```python
from build123d import *

# Parameters (mm, degrees)
CROQUIS1_R              = 5
SALIENTE_EXTRUIR1_DEPTH = 40
CORTAR_EXTRUIR2_DEPTH   = 10
CORTAR_EXTRUIR4_DEPTH   = 20
CROQUIS6_R              = 12.2
CORTAR_EXTRUIR6_DEPTH   = 63
CORTAR_EXTRUIR9_DEPTH   = 30
CROQUIS8_W              = 12.2
CROQUIS8_H              = 11.6
CORTAR_EXTRUIR10_DEPTH  = 66
CORTAR_EXTRUIR11_REACH  = 151.27
CROQUIS9_W              = 11.6
CROQUIS9_H              = 11.6
CHAFL_N1_SIZE           = 10


with BuildPart() as part:
    # Croquis1 → Saliente-Extruir1 (new body)
    with BuildSketch(Plane.XY):
        with BuildLine():
            Line((106.972889038, 33), (-43.027110962, 33))
            ThreePointArc((-43.027110962, 33), (-76.027110962, 0), (-43.027110962, -33))
            Line((-43.027110962, -33), (106.972889038, -33))
            ThreePointArc((106.972889038, -33), (139.972889038, 0), (106.972889038, 33))
        make_face()
        with Locations((106.972889038, 0)):
            Circle(CROQUIS1_R, mode=Mode.SUBTRACT)
    extrude(amount=SALIENTE_EXTRUIR1_DEPTH)

    # Croquis1<4> → Cortar-Extruir2 (cut)
    with BuildSketch(Plane.XY):
        with BuildLine():
            Line((-41.509889959, -1.303088803), (-41.509889959, 1.303088803))
            ThreePointArc((-41.509889959, 1.303088803), (-45.027110962, 0), (-41.509889959, -1.303088803))
        make_face()
    extrude(amount=CORTAR_EXTRUIR2_DEPTH, mode=Mode.SUBTRACT)

    # Croquis5 → Cortar-Extruir4 (cut)
    with BuildSketch(Plane.XY.offset(40)):
        Polygon((96.972889038, -12.2), (96.972889038, 12.2), (33.972889038, 12.2), (33.972889038, -23.8), (42.805927542, -23.8), (42.805927542, -12.2), align=None)
    extrude(amount=-CORTAR_EXTRUIR4_DEPTH, mode=Mode.SUBTRACT)

    # Croquis6 → Cortar-Extruir6 (cut)
    with BuildSketch(Plane(origin=(33.972889038, 0, 0), x_dir=(0, 0, -1), z_dir=(1, 0, 0))):
        with Locations((-20, 0)):
            Circle(CROQUIS6_R)
        with BuildLine():
            ThreePointArc((-20, -12.2), (-32.2, 0), (-20, 12.2))
            Line((-20, 12.2), (-40, 12.2))
            Line((-40, 12.2), (-40, -12.2))
            Line((-40, -12.2), (-20, -12.2))
        make_face()
    extrude(amount=CORTAR_EXTRUIR6_DEPTH, mode=Mode.SUBTRACT)

    # Croquis7 → Cortar-Extruir9 (cut)
    with BuildSketch(Plane.ZY.offset(-96.972889038)):
        with BuildLine():
            ThreePointArc((7.8, -3.1e-08), (11.37329728, -8.626702741), (20, -12.2))
            Line((20, -12.2), (32.2, -12.2))
            Line((32.2, -12.2), (32.2, 12.2))
            Line((32.2, 12.2), (20, 12.2))
            ThreePointArc((20, 12.2), (11.373297259, 8.62670272), (7.8, -3.1e-08))
        make_face()
        with BuildLine():
            Line((7.8, -12.2), (20, -12.2))
            ThreePointArc((20, -12.2), (11.37329728, -8.626702741), (7.8, -3.1e-08))
            Line((7.8, -3.1e-08), (7.8, -12.2))
        make_face()
        with BuildLine():
            Line((7.8, 12.2), (7.8, -3.1e-08))
            ThreePointArc((7.8, -3.1e-08), (11.373297259, 8.62670272), (20, 12.2))
            Line((20, 12.2), (7.8, 12.2))
        make_face()
    extrude(amount=-CORTAR_EXTRUIR9_DEPTH, mode=Mode.SUBTRACT)

    # Croquis8 → Cortar-Extruir10 (cut)
    with BuildSketch(Plane(origin=(33.972889038, 0, 0), x_dir=(0, 0, -1), z_dir=(1, 0, 0))):
        with Locations((-26.1, -18)):
            Rectangle(CROQUIS8_W, CROQUIS8_H)
    extrude(amount=-CORTAR_EXTRUIR10_DEPTH, mode=Mode.SUBTRACT)

    # Croquis9 → Cortar-Extruir11 (cut, up to next)
    with BuildSketch(Plane(origin=(0, 0, 0), x_dir=(-1, 0, 0), z_dir=(0, 0, -1)), mode=Mode.PRIVATE) as cortar_extruir11_sk1:
        with Locations((26.227110962, -18)):
            Rectangle(CROQUIS9_W, CROQUIS9_H)
    cortar_extruir11_tool1 = extrude(cortar_extruir11_sk1.sketch, amount=-CORTAR_EXTRUIR11_REACH, mode=Mode.PRIVATE) & part.part
    add(cortar_extruir11_tool1.solids().sort_by_distance((-26.227111, -18, 0))[0], mode=Mode.SUBTRACT)

    # Chaflán1
    chafl_n1_edges = [part.edges().sort_by_distance(p)[0] for p in [
        (-32.027110962, -18, 0),
    ]]
    chamfer(chafl_n1_edges, length=CHAFL_N1_SIZE)


solid = part.part
```
Could you check a few things on this model? Use its own coordinates, in mm. A direction names the side the tool comes from. Give positions to 0.01 mm unless a question says otherwise; leave off trailing zeros. Loops run counter-clockwise (first coordinate to the right, second up) from the corner with the lowest first, then second, coordinate; pieces in that order, holes last. Notation, with made-up numbers: (10, 76) - (52, 76) arc R9 ccw to (52, 83) - close; hole circle Ø10 at (58, 4.25). An arc over 180 degrees is marked (long way). Answer in a Markdown table with one row per item. Add a question column.
Q1. If we section it at D-D (x = -63): List the corners of the cut face in (y, z) for me, plus the area to 3 significant figures.
Q2. If we section it at C-C (x = 122): List the corners of the cut face in (y, z) for me.
Q3. Please list where these lines run through material, in increasing order: L1, parallel to X at y = 0, z = 3; L2, parallel to X at y = 0, z = 38; L3, parallel to Y at x = 71.5, z = 32. Write a range as from..to.
Q4. If we section it at B-B (z = 29): List the corners of the cut face in (x, y) for me, plus the area to 3 significant figures.
Q5. Which directions (+Z, -Z, +X, -X, +Y, -Y) give clear straight access to the entire face, cutting with the end or side of a thin tool? Please do faces 1 (the face through (65.032, -0.268, 7.803)), 2 (the face through (-37.097, -18.081, 4.93)), 3 (the face through (96.973, -9, 10)).
Q6. If we section it at A-A (x = 32): List the corners of the cut face in (y, z) for me.
Q7. We'd pull the mould along Y, two halves only. Please class faces 4 (the face through (30, 0, 0)), 5 (the face through (84, -12.2, 28)), 6 (the face through (139.965, -0.726, 19.72)), 7 (the face through (111.59, -1.92, 3.85)): +Y half, -Y half, draft (parallel to the pull), parting line (faces both ways), or undercut.
Q8. For pin 1 (3 mm diameter, centred on y = 0, z = 3, fed in from -X); pin 2 (4 mm diameter, centred on y = -20.5, z = 23, fed in from +X); pin 3 (2.5 mm diameter, centred on y = -5.5, z = 37, fed in from -X), each with a flat end and sliding along its axis, tell me the tip position at first contact or that it passes through.
The answers:
| question | item | result |
|---|---|---|
| 1 | outline | (-26.27, 0) - (26.27, 0) - (26.27, 40) - (-26.27, 40) - close |
| 1 | area | 2,100 mm^2 |
| 2 | outline | (-29.38, 0) - (29.38, 0) - (29.38, 40) - (-29.38, 40) - close; hole (-12.2, 7.8) - (12.2, 7.8) - (12.2, 32.2) - (-12.2, 32.2) - close |
| 3 | L1 | x = -76.03..-45.03, -41.51..101.97, 111.97..139.97 |
| 3 | L2 | x = -76.03..33.97, 96.97..101.97, 111.97..139.97 |
| 3 | L3 | y = -33..-12.2, 12.2..33 |
| 4 | outline | (-43.03, -33) - (106.97, -33) arc R33 ccw to (106.97, 33) - (-43.03, 33) arc R33 ccw to start; hole (-32.03, -23.8) - (42.81, -23.8) - (42.81, -12.2) - (126.97, -12.2) - (126.97, 12.2) - (33.97, 12.2) - (33.97, -12.2) - (-32.03, -12.2) - close |
| 4 | area | 10,200 mm^2 |
| 5 | face 1 | +Z |
| 5 | face 2 | -Z |
| 5 | face 3 | none |
| 6 | outline | (-33, 0) - (33, 0) - (33, 40) - (-33, 40) - close; hole (-23.8, 20) - (-12.2, 20) - (-12.2, 32.2) - (-23.8, 32.2) - close |
| 7 | face 4 | draft |
| 7 | face 5 | undercut |
| 7 | face 6 | parting line |
| 7 | face 7 | undercut |
| 8 | pin 1 | stops at x = -76.03 |
| 8 | pin 2 | stops at x = 134.3 |
| 8 | pin 3 | stops at x = -75.75 |
